Autodesk Inventor part; units mm, degrees
ref_plane "YZ Plane" through (0, 0, 0) normal (1, 0, 0) x (0, 1, 0)
ref_plane "XZ Plane" through (0, 0, 0) normal (0, 1, 0) x (-1, 0, 0)
ref_plane "XY Plane" through (0, 0, 0) normal (0, 0, 1) x (1, 0, 0)
sketch "Sketch1" plane through (0, 0, 0) normal (0, 1, 0) x (-1, 0, 0)
  line L0 (0, 0) -> (60, 0)
  line L1 (60, 0) -> (60, -110)
  line L2 (60, -110) -> (0, -110)
  line L3 (0, -110) -> (0, 0)
  dimension "d0" = 110
  dimension "d1" = 60
sketch "Sketch2" plane through (0, 0, 0) normal (0, 1, 0) x (-1, 0, 0)
  line L0 (1.1114, -30.6908) -> (-33.2555, -30.6908)
  line L1 (-33.2555, -30.6908) -> (-33.2555, -38.7269)
  line L2 (-33.2555, -38.7269) -> (1.1114, -38.7269)
  line L3 (1.1114, -38.7269) -> (1.1114, -30.6908)
  line L4 (1.1114, -46.079) -> (-33.2555, -46.079)
  line L5 (-33.2555, -46.079) -> (-33.2555, -53.9441)
  line L6 (-33.2555, -53.9441) -> (1.1114, -53.9441)
  line L7 (1.1114, -53.9441) -> (1.1114, -46.079)
  line L8 (1.1114, -61.8091) -> (-33.2555, -61.8091)
  line L9 (-33.2555, -61.8091) -> (-33.2555, -69.1613)
  line L10 (-33.2555, -69.1613) -> (1.1114, -69.1613)
  line L11 (1.1114, -69.1613) -> (1.1114, -61.8091)
  line L12 (1.1114, -75.4875) -> (-33.2555, -75.4875)
  line L13 (-33.2555, -75.4875) -> (-33.2555, -83.0106)
  line L14 (-33.2555, -83.0106) -> (1.1114, -83.0106)
  line L15 (1.1114, -83.0106) -> (1.1114, -75.4875)
  point P0 (0, 0)
extrude "Extrusion1" add sketch "Sketch1" along normal blind 10
extrude "Extrusion2" add sketch "Sketch2" against normal blind 3
sketch "Sketch3" plane through (0, 10, 0) normal (0, 1, 0) x (1, 0, 0)
  circle A0 centre (-29.665, 24.7066) radius 18.0252
  circle A1 centre (-29.665, 81.1298) radius 18.0284
  point P0 (0, 0)
extrude "Extrusion3" add sketch "Sketch3" along normal blind 10
sketch "Sketch4" plane through (-29.665, 20, -24.7066) normal (0, 1, 0) x (1, 0, 0)
  point P0 (29.665, -24.7066)
sketch "Sketch5" plane through (-29.665, 20, -24.7066) normal (0, 1, 0) x (1, 0, 0)
  circle A0 centre (0, 0) radius 18.0252
  point P0 (29.665, -24.7066)
hole "Hole1" at (-29.665, 20, -24.7066) direction (0, -1, 0) diameter 30 depth 3
sketch "Sketch6" plane through (-29.665, 20, -81.1298) normal (0, 1, 0) x (1, 0, 0)
  circle A0 centre (0, 0) radius 18.0284
  point P0 (29.665, -81.1298)
hole "Hole2" at (-29.665, 20, -81.1298) direction (0, -1, 0) diameter 30 depth 3
sketch "Sketch7" plane through (0, 10, 0) normal (0, 1, 0) x (1, 0, 0)
  point P0 (0, 0)
  point P1 (-54.5256, 5.8465)
  point P2 (-54.9391, 103.1409)
  point P3 (-6.5559, 103.7715)
  point P4 (-5.4452, 5.4602)
hole "Hole3" at (-54.5256, 10, -5.8465) at (-54.9391, 10, -103.1409) at (-6.5559, 10, -103.7715) at (-5.4452, 10, -5.4602) direction (0, -1, 0) diameter 8 end through all
sketch "Sketch8" plane through (0, 10, 0) normal (0, 1, 0) x (1, 0, 0)
  line L0 (-57.5346, 24.8775) -> (-57.5346, 80.9707) construction
  line L1 (-57.5346, 80.9707) -> (-48.1627, 80.9707) construction
  line L2 (-48.1627, 80.9707) -> (-48.1627, 24.8775) construction
  line L3 (-48.1627, 24.8775) -> (-57.5346, 24.8775) construction
  point P0 (0, 0)
properties part number "ultrasonic now"
Geometry check sheet. Reference: the model listing, model coordinates, mm. A direction names the side the tool comes from. Coordinates: 2 decimals unless noted, no trailing zeros. Order: outer loops, then holes, each group sorted by start corner. A loop starts at its lowest first (then second) coordinate and runs counter-clockwise, first axis right, second up. Notation, with made-up numbers: M 1.5,86.25 L 56.5,86.25 A19 cw 56.5,118.25 Z; hole C 23,32 d5. An arc over 180 degrees is marked long. One line per question, with ' | ' between items. Start each with the question number.
Item 1: Cross-section at A-A on x = 12. Enter the section's corners in (y, z).
Item 2: Set-up check for faces 4 (the flat face through (-1.111, -1, -79)), 5 (the cylindrical face through (-33.573, 14.93, -42.303)), 6 (the flat face through (0, 5, -56)), 7 (the flat face through (-60, 5, -54)): record each of +Z, -Z, +X, -X, +Y, -Y from which the full face is reachable in a straight line by a thin tool's end or side.
Item 3: Cross-section at D-D on x = -18.5. Enter the section's corners in (y, z), then the cut area to 3 significant figures.
Item 4: Material ranges on L1, parallel to X at y = 6.5, z = -5 (3 decimals); L2, parallel to Y at x = -13, z = -75; L3, parallel to Y at x = -25, z = -86, recorded low to high. Write a range as [from, to].
Item 5: Draft check along X on faces 1 (the flat face through (-1.111, -1, -66)), 2 (the cylindrical face through (-3.913, 4.93, -1.765)), 3 (the flat face through (33.256, -1, -65)). Enter one of: pulls with the +X half, pulls with the -X half, needs draft (parallel to the pull), parting line crosses it, or undercut.
Item 6: Gauge pin test, flat ends, axial feed: pin 1 (10.5 mm diameter, centred on x = -54.53, z = -5.85, fed in from -Y); pin 2 (8 mm diameter, centred on x = -5, z = -39, fed in from +Y); pin 3 (8.5 mm diameter, centred on x = 8.5, z = -50, fed in from +Y); pin 4 (5 mm diameter, centred on x = -5.45, z = -5.46, fed in from -Y). Record the tip position at first contact, or that the pin passes through.
Item 7: Cross-section at B-B on z = -52.5. Enter the section's corners in (x, y), then the cut area to 3 significant figures.
Item 8: Cross-section at C-C on y = 7.5. Enter the section's corners in (x, z), then the cut area to 3 significant figures.
Findings:
1) outline: M -3,-83.01 L 0,-83.01 L 0,-75.49 L -3,-75.49 Z; M -3,-69.16 L 0,-69.16 L 0,-61.81 L -3,-61.81 Z; M -3,-53.94 L 0,-53.94 L 0,-46.08 L -3,-46.08 Z; M -3,-38.73 L 0,-38.73 L 0,-30.69 L -3,-30.69 Z
2) face 4: +Z, -Z, -X, -Y | face 5: +Y | face 6: +Z, -Z, +X, +Y | face 7: +Z, -Z, -X, +Y, -Y
3) outline: M 0,-110 L 10,-110 L 10,-95.28 L 20,-95.28 L 20,-91.15 L 17,-91.15 L 17,-71.11 L 20,-71.11 L 20,-66.97 L 10,-66.97 L 10,-38.86 L 20,-38.86 L 20,-34.72 L 17,-34.72 L 17,-14.69 L 20,-14.69 L 20,-10.56 L 10,-10.56 L 10,0 L 0,0 Z | area: 1,550 mm²
4) L1: x = [-60, -58.435], [-50.616, -9.419], [-1.472, 0] | L2: y = [0, 20] | L3: y = [0, 17]
5) face 1: pulls with the -X half | face 2: undercut | face 3: pulls with the +X half
6) pin 1: stops at y = 0 | pin 2: stops at y = 10 | pin 3: stops at y = 0 | pin 4: passes through
7) outline: M -60,0 L -1.11,0 L -1.11,-3 L 33.26,-3 L 33.26,0 L 0,0 L 0,10 L -60,10 Z | area: 703 mm²
8) outline: M -60,-110 L 0,-110 L 0,0 L -60,0 Z; hole C -54.94,-103.14 d8; hole C -54.53,-5.85 d8; hole C -6.56,-103.77 d8; hole C -5.45,-5.46 d8 | area: 6,400 mm²
